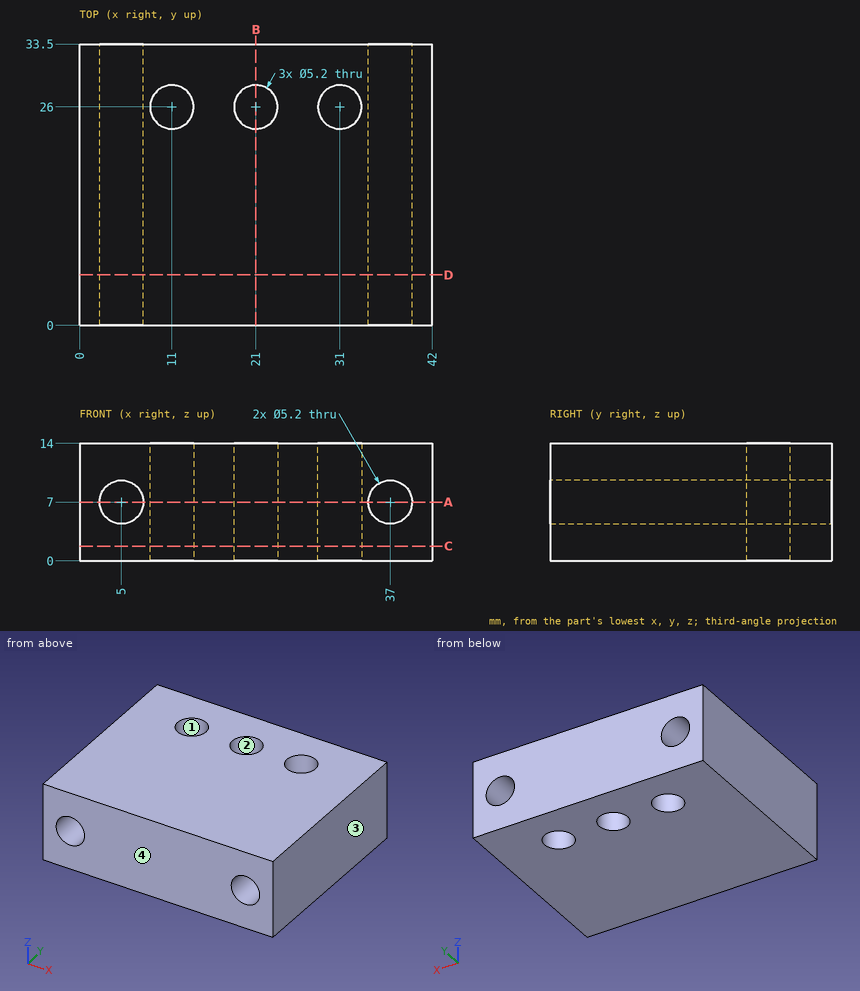
Job drawing, mm, ordinate dimensions from the low corner. One solid piece. Coordinates: 2 decimals unless noted, no trailing zeros. Loops run counter-clockwise (first coordinate to the right, second up) from the corner with the lowest first, then second, coordinate; pieces in that order, holes last. Notation, with made-up numbers: (-8, 63) - (21, 63) arc R20 ccw to (21, 93) - close; hole circle Ø6 at (-39, 54.25). An arc over 180 degrees is marked (long way). Answer as a JSON object with one key per item and string values. Group by question number.
(1) Probe line 1 along X through (y, z) = (9, 7); line 2 along X through (y, z) = (25.5, 7.5); line 3 along Y through (x, z) = (31, 4.25). List the from-to ranges inside material, lowest first.
(2) Cut at C-C (z = 1.75). Give the cut face in (x, y), then the cut area to 3 significant figures.
(3) Cut at D-D (y = 6). Give the cut face in (x, z), then the cut area to 3 significant figures.
(4) Cut at A-A (z = 7). Give the cut face in (x, y).
(5) Two-plate mould, pull along X, no slides. Class the marked faces 1, 2, 3 and 4: released by +X, released by -X, zero draft, split by the parting line, or undercut.
(6) Cut at B-B (x = 21). Give the cut face in (y, z), then the cut area to 3 significant figures.
Geometry says:
{
 "1": {"line 1": "x = 0 to 2.4, 7.6 to 34.4, 39.6 to 42", "line 2": "x = 0 to 2.45, 7.55 to 8.45, 13.55 to 18.45, 23.55 to 28.45, 33.55 to 34.45, 39.55 to 42", "line 3": "y = 0 to 23.4, 28.6 to 33.5"},
 "2": {"outline": "(0, 0) - (42, 0) - (42, 33.5) - (0, 33.5) - close; hole circle Ø5.2 at (11, 26); hole circle Ø5.2 at (21, 26); hole circle Ø5.2 at (31, 26)", "area": "1,340 mm^2"},
 "3": {"outline": "(0, 0) - (42, 0) - (42, 14) - (0, 14) - close; hole circle Ø5.2 at (5, 7); hole circle Ø5.2 at (37, 7)", "area": "546 mm^2"},
 "4": {"outline": "(0, 0) - (2.4, 0) - (2.4, 33.5) - (0, 33.5) - close; (7.6, 0) - (34.4, 0) - (34.4, 33.5) - (7.6, 33.5) - close; (39.6, 0) - (42, 0) - (42, 33.5) - (39.6, 33.5) - close; hole circle Ø5.2 at (11, 26); hole circle Ø5.2 at (21, 26); hole circle Ø5.2 at (31, 26)"},
 "5": {"face 1": "undercut", "face 2": "undercut", "face 3": "released by +X", "face 4": "zero draft"},
 "6": {"outline": "(0, 0) - (23.4, 0) - (23.4, 14) - (0, 14) - close; (28.6, 0) - (33.5, 0) - (33.5, 14) - (28.6, 14) - close", "area": "396 mm^2"}
}
